Autodesk Inventor part; units mm, degrees
ref_plane "YZ Plane" through (0, 0, 0) normal (1, 0, 0) x (0, 1, 0)
ref_plane "XZ Plane" through (0, 0, 0) normal (0, 1, 0) x (-1, 0, 0)
ref_plane "XY Plane" through (0, 0, 0) normal (0, 0, 1) x (1, 0, 0)
sketch "Skizze1" plane through (0, 0, 0) normal (0, 0, 1) x (1, 0, 0)
  line L0 (0, 0) -> (0, 12)
  line L1 (0, 12) -> (12, 12)
  line L2 (12, 12) -> (12, 9.5)
  line L3 (12, 9.5) -> (17.9, 9.5)
  line L4 (17.9, 9.5) -> (17.9, 5)
  line L5 (0, 0) -> (17.1, 0)
  line L6 (17.9, 5) -> (17.1, 5)
  line L7 (17.1, 5) -> (17.1, 0)
  dimension "d0" = 19
  dimension "d1" = 24
  dimension "d2" = 5.9
  dimension "d3" = 12
  dimension "d12" = 10
  dimension "d13" = 5.1
revolve "Umdrehung1" add sketch "Skizze1" angle 360 about axis through (0, 0, 0) along (1, 0, 0)
sketch "Skizze2" plane through (0, 0, 0) normal (-1, 0, 0) x (0, 0, 1)
  point P0 (0, 0)
  point P1 (0, 0)
hole "Bohrung1" at (0, 0, 0) direction (1, 0, 0) diameter 4.134 end through all
feature "Verdickung1" [suppressed]
thicken "Verdickung2" operation add thickness 0.1 both sides no extend neighbours yes toward (0, 0.9870503, -0.1604113) faces at (17.3667, 4.9353, -0.8021)
properties part number "SpringCompensation_Outside_DrivenPart"
CAD build for the part. Positions are in the model's coordinates, mm. A direction names the side the tool comes from. Coordinates: 2 decimals unless noted, no trailing zeros. Order: outer loops, then holes, each group sorted by start corner. A loop starts at its lowest first (then second) coordinate and runs counter-clockwise, first axis right, second up.
Item 1: Band-saw the part on C-C on x = 13. List the corners of the cut face in (y, z), plus the area to 3 significant figures.
Check sheet entries:
outline: circle Ø19 at (0, 0); hole circle Ø4.13 at (0, 0)
area: 270 mm2
Item 2: Two-plate mould, pull along Y, no slides. Class faces 3 (the face through (17.5, 2.4, 4.5)), 4 (the face through (0, 2.5, 0.2)), 5 (the face through (6.08, -11.99, 0.53)): +Y half, -Y half, draft (parallel to the pull), parting line (faces both ways), or undercut.
Check sheet entries:
face 3: undercut
face 4: draft
face 5: parting line
Item 3: Pin check, flat tips, straight feed: pin 1 Ø10 at (y, z) = (4, 4.5) entering from -X; pin 2 Ø10 at (x, z) = (15.5, -7.5) entering from +Y; pin 3 Ø9 at (y, z) = (0, 0) entering from +X; pin 4 Ø1.5 at (x, y) = (6, -8) entering from +Z. Stop position of each tip, or through.
Check sheet entries:
pin 1: stops at x = 0
pin 2: stops at y = 11.34
pin 3: stops at x = 17.1
pin 4: stops at z = 9.56
Item 4: Band-saw the part on A-A on z = 0. List the corners of the cut face in (x, y), plus the area to 3 significant figures.
Check sheet entries:
outline: (0, -12) - (12, -12) - (12, -9.5) - (17.9, -9.5) - (17.9, -5.1) - (17.1, -5.1) - (17.1, -2.07) - (0, -2.07) - close; (0, 2.07) - (17.1, 2.07) - (17.1, 5.1) - (17.9, 5.1) - (17.9, 9.5) - (12, 9.5) - (12, 12) - (0, 12) - close
area: 321 mm2
Item 5: Band-saw the part on D-D on z = -2.75. List the corners of the cut face in (x, y), plus the area to 3 significant figures.
Check sheet entries:
outline: (0, -11.68) - (12, -11.68) - (12, -9.09) - (17.9, -9.09) - (17.9, -4.3) - (17.1, -4.3) - (17.1, 4.3) - (17.9, 4.3) - (17.9, 9.09) - (12, 9.09) - (12, 11.68) - (0, 11.68) - close
area: 381 mm2
Item 6: Drill centre lines: L1, parallel to Z at x = 17.5, y = 0; L2, parallel to Z at x = 10.25, y = 0; L3, parallel to X at y = -6.5, z = 9.5. Where is each one in solid material? Low to high.
Check sheet entries:
L1: z = -9.5 to -5.1, 5.1 to 9.5
L2: z = -12 to -2.07, 2.07 to 12
L3: x = 0 to 12
Item 7: 3-axis set-ups, long thin cutter, end or side, ignore diameter. For faces 1 (the face through (17.9, 4, -4)), 2 (the face through (14.99, 4.38, -8.43)): which of +Z, -Z, +X, -X, +Y, -Y reach the whole face in a straight line?
Check sheet entries:
face 1: +Z, -Z, +X, +Y, -Y
face 2: +X
